Model file for the job. Use its own axes, mm. A direction names the side the tool comes from. Coordinates: 2 decimals unless noted, no trailing zeros. Write each loop counter-clockwise with the first axis right and the second up, starting at its lowest first coordinate (ties: lowest second). Pieces come first, ordered by that corner, then holes. Notation, with made-up numbers: M 52.5,-39 L 104.5,-39 A22 ccw 104.5,-19 Z; hole C -2,20.25 d7. An arc over 180 degrees is marked long. Put each result on its own line as item: value. Start each with the question number.
Q1. Drop flat-ended pins along their axis: pin 1 (6 mm diameter, centred on y = -9, z = 9.5, fed in from -X); pin 2 (9 mm diameter, centred on x = -32.5, z = 8, fed in from -Y); pin 3 (8 mm diameter, centred on x = -13, z = 3, fed in from +Y). Give the stop position or say it passes through.
Q2. Drill centre lines: line 1 along X through (y, z) = (46, 5); line 2 along X through (y, z) = (-21, 7); line 3 along X through (y, z) = (28, 3.25). Where is each one in solid material? Low to high.
Q3. Cut at C-C (x = -11). Write the cut outline in (y, z).
Q4. Which spindle directions (+Z, -Z, +X, -X, +Y, -Y) get a long thin tool onto all of the face, cutting with end or side? Do faces 1 (the flat face through (0, 25.202, 9)), 2 (the flat face through (28, 13.664, 9)), 3 (the flat face through (-28.391, 37, 9)). Say none if no direction does.
Q5. Pull direction X, two halves, no side cores. Call faces 4 (the flat face through (-42.662, 32, 9)), 5 (the flat face through (-28, 13.664, 9)), 6 (the flat face through (28.391, 37, 9)), 7 (the cylindrical face through (14.961, 12.136, 9.014)): pulls with the +X half, pulls with the -X half, needs draft (parallel to the pull), parting line crosses it, or undercut.
Q6. Cut at B-B (z = 2.5). Write the cut outline in (x, y).
Q7. Cut at D-D (y = 2.5). Write the cut outline in (x, z).
Q8. Cut at A-A (y = 43). Write the cut outline in (x, z), then the cut area to 3 significant figures.
```python
from build123d import *

# Parameters (mm, degrees)
F1_DEPTH = 17.78
F2_R     = 5.08
F3_R     = 12.877415


with BuildPart() as f1:
    # F0 (on Top) → F1 (new body)
    with BuildSketch(Plane.XY):
        with BuildLine():
            Line((-13.512124, -44.939205), (0, -44.939205))
            Line((0, -44.939205), (13.512124, -44.939205))
            Line((13.512124, -44.939205), (13.512124, 13.663948))
            Line((13.512124, 13.663948), (42.661879, 13.663948))
            Line((42.661879, 13.663948), (42.661879, 44.331919))
            ThreePointArc((42.661879, 44.331919), (35.526263, 54.048505), (28.390646, 44.331919))
            Line((28.390646, 44.331919), (28.390646, 25.202392))
            Line((28.390646, 25.202392), (0, 25.202392))
            Line((0, 25.202392), (-28.390646, 25.202392))
            Line((-28.390646, 25.202392), (-28.390646, 44.331919))
            ThreePointArc((-28.390646, 44.331919), (-35.526263, 54.048505), (-42.661879, 44.331919))
            Line((-42.661879, 44.331919), (-42.661879, 13.663948))
            Line((-42.661879, 13.663948), (-13.512124, 13.663948))
            Line((-13.512124, 13.663948), (-13.512124, -44.939205))
        make_face()
    extrude(amount=F1_DEPTH)

    # F2
    f2_edges = [f1.edges().sort_by_distance(p)[0] for p in [
        (-42.661879, 13.663948, 8.89),
        (-13.512124, 13.663948, 8.89),
        (42.661879, 13.663948, 8.89),
        (13.512124, 13.663948, 8.89),
        (28.390646, 25.202392, 8.89),
        (-28.390646, 25.202392, 8.89),
    ]]
    fillet(f2_edges, radius=F2_R)

    # F3
    f3_edges = [f1.edges().sort_by_distance(p)[0] for p in [
        (-13.512124, -44.939205, 8.89),
        (13.512124, -44.939205, 8.89),
    ]]
    fillet(f3_edges, radius=F3_R)


solid = f1.part
```
Computed values:
1. pin 1: x = -13.51
1. pin 2: y = 13.66
1. pin 3: y = 25.2
2. line 1: -42.98 to -28.07, 28.07 to 42.98
2. line 2: -13.51 to 13.51
2. line 3: -42.66 to -27.85, 27.85 to 42.66
3. outline: M -39.7,0 L 25.2,0 L 25.2,17.78 L -39.7,17.78 Z
4. face 1: +Z, -Z, +Y
4. face 2: +Z, -Z, +X, -Y
4. face 3: +Z, -Z
5. face 4: pulls with the -X half
5. face 5: needs draft
5. face 6: undercut
5. face 7: pulls with the +X half
6. outline: M -42.66,18.74 A5.08 ccw -37.58,13.66 L -18.59,13.66 A5.08 cw -13.51,8.58 L -13.51,-32.06 A12.88 ccw -0.63,-44.94 L 0.63,-44.94 A12.88 ccw 13.51,-32.06 L 13.51,8.58 A5.08 cw 18.59,13.66 L 37.58,13.66 A5.08 ccw 42.66,18.74 L 42.66,44.33 A7.48 ccw long 28.39,44.33 L 28.39,30.28 A5.08 cw 23.31,25.2 L -23.31,25.2 A5.08 cw -28.39,30.28 L -28.39,44.33 A7.48 ccw long -42.66,44.33 Z
7. outline: M -13.51,0 L 13.51,0 L 13.51,17.78 L -13.51,17.78 Z
8. outline: M -42.66,0 L -28.39,0 L -28.39,17.78 L -42.66,17.78 Z; M 28.39,0 L 42.66,0 L 42.66,17.78 L 28.39,17.78 Z
8. area: 507 mm2
